Could you check a few things on this drawing? It's one solid part, dimensions in mm from its lowest x, y, z. Round coordinates to 2 decimals unless told otherwise and drop trailing zeros. Order: outer loops, then holes, each group sorted by start corner. A loop starts at its lowest first (then second) coordinate and runs counter-clockwise, first axis right, second up. Notation, with made-up numbers: (-24, -39) - (-16, -39) arc R17 cw to (-16, -16) - close; hole circle Ø4 at (88.25, -23.5). An arc over 180 degrees is marked (long way). Use one line per item in the form item = value.
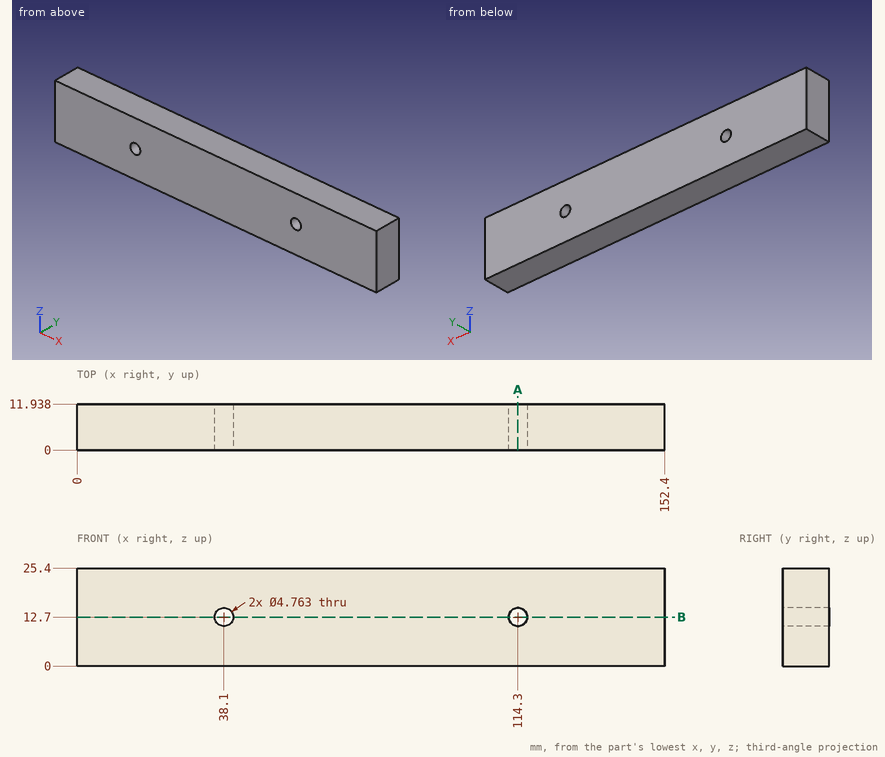
Item 1: Imagine slicing it at B-B on z = 12.7. Please give me the cut outline in (x, y).
Found:
outline = (0, 0) - (35.72, 0) - (35.72, 11.94) - (0, 11.94) - close; (40.48, 0) - (111.92, 0) - (111.92, 11.94) - (40.48, 11.94) - close; (116.68, 0) - (152.4, 0) - (152.4, 11.94) - (116.68, 11.94) - close
Item 2: Will this pin go through, and if not, where does the flat tip stop? P1, Ø4.5, axis at x = 38.1, z = 12.7, coming from the +Y side.
Found:
P1 = through
Item 3: Imagine slicing it at A-A on x = 114.3. Please give me the cut outline in (y, z).
Found:
outline = (0, 0) - (11.94, 0) - (11.94, 10.32) - (0, 10.32) - close; (0, 15.08) - (11.94, 15.08) - (11.94, 25.4) - (0, 25.4) - close
Item 4: I need wall thicknesses on L1, parallel to X at y = 5.25, z = 11.25; L2, parallel to X at y = 8.5, z = 14.25; L3, parallel to Z at x = 38.1, y = 6.25. Which ranges of each line are inside material? Lowest first, please.
Found:
L1 = 0 to 36.21, 39.99 to 112.41, 116.19 to 152.4
L2 = 0 to 36.29, 39.91 to 112.49, 116.11 to 152.4
L3 = 0 to 10.32, 15.08 to 25.4
